Input: part model. Units: mm. Frame: model coordinates. Face numbers are marked on the shaded views. A direction names the side the tool comes from. Give positions to 0.01 mm unless a question says otherwise; leave off trailing zeros. Order: outer loops, then holes, each group sorted by start corner. A loop starts at its lowest first (then second) coordinate and runs counter-clockwise, first axis right, second up.
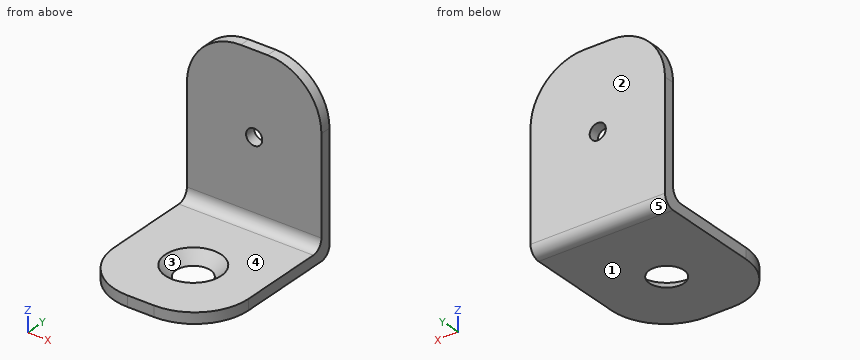
```python
from build123d import *

# Parameters (mm, degrees)
EXTRUDE_1_DEPTH     = 2
EXTRUDE_2_DEPTH     = 2
FILLET_1_R          = 2
FILLET_2_R          = 2
SKETCH_8_R          = 1.5
CUT_EXTRUDE_1_DEPTH = 10


with BuildPart() as part:
    # Эскиз1 → Бобышка-Вытянуть1 (new body)
    with BuildSketch(Plane(origin=(0, 0, 0), x_dir=(1, 0, 0), z_dir=(0, 1, 0))):
        with BuildLine():
            Line((-2.5, -15), (2.5, -15))
            ThreePointArc((2.5, -15), (9.571067812, -12.071067812), (12.5, -5))
            Line((12.5, -5), (12.5, 15))
            Line((12.5, 15), (-12.5, 15))
            Line((-12.5, 15), (-12.5, -5))
            ThreePointArc((-12.5, -5), (-9.571067812, -12.071067812), (-2.5, -15))
        make_face()
    extrude(amount=EXTRUDE_1_DEPTH)

    # Эскиз3 → Бобышка-Вытянуть2 (add)
    with BuildSketch(Plane(origin=(0, 0, -15), x_dir=(-1, 0, 0), z_dir=(0, 0, -1))):
        with BuildLine():
            Line((-2.5, -28), (2.5, -28))
            ThreePointArc((2.5, -28), (9.571067812, -25.071067812), (12.5, -18))
            Line((12.5, -18), (12.5, 2))
            Line((12.5, 2), (-12.5, 2))
            Line((-12.5, 2), (-12.5, -18))
            ThreePointArc((-12.5, -18), (-9.571067812, -25.071067812), (-2.5, -28))
        make_face()
    extrude(amount=EXTRUDE_2_DEPTH)

    # Скругление1
    fillet_1_edges = [part.edges().sort_by_distance(p)[0] for p in [
        (0, 0, -15),
    ]]
    fillet(fillet_1_edges, radius=FILLET_1_R)

    # Скругление2
    fillet_2_edges = [part.edges().sort_by_distance(p)[0] for p in [
        (0, 2, -17),
    ]]
    fillet(fillet_2_edges, radius=FILLET_2_R)

    # Эскиз7 → Зенковка для винта с полупотайной головкой M52 (revolve, cut)
    with BuildSketch(Plane(origin=(0, -15.034247801, -15), x_dir=(0, -1, 0), z_dir=(1, 0, 0))):
        Polygon((0, 0), (0, 2), (2.75, 2), (2.75, 2.45), (5.2, 0), align=None)
    revolve(axis=Axis((0, -15.034247801, -8.65), (0, 0, -1)), mode=Mode.SUBTRACT)

    # Эскиз8 → Вырез-Вытянуть1 (cut)
    with BuildSketch(Plane.XZ):
        Circle(SKETCH_8_R)
    extrude(amount=-CUT_EXTRUDE_1_DEPTH, mode=Mode.SUBTRACT)


solid = part.part
```
1) Reachability of the marked faces 4 and 5 from +Z, -Z, +X, -X, +Y, -Y: full face, straight path, thin tool, end or side. Return the list, or none.
2) Cut plane B-B (x = 8.5). Return the cut outline in (y, z), then the cut area to 3 significant figures.
3) Cut plane A-A (z = 0). Return the cut outline in (x, y).
4) Line query: probe 1 along Y at (x, z) = (6.75, 12); probe 2 along Z at (x, y) = (8, -13); probe 3 along Z at (x, y) = (0, 1.2). Output: solid intervals per line, ascending.
5) Cut plane D-D (x = -6). Return the cut outline in (y, z), then the cut area to 3 significant figures.
6) Cut plane C-C (z = -7.5). Return the cut outline in (x, y), then the cut area to 3 significant figures.
7) First-contact query: P1, Ø10, axis at x = 4.5, z = -7, coming from the -Y side; P2, Ø1.8, axis at x = 0, z = 0, coming from the -Y side; P3, Ø12.5, axis at x = 2, y = -18, coming from the +Z side. Flat tips, straight axial feed; report the tip coordinate or a pass-through.
8) Pull-direction query (Y, two-part tool) for the marked faces 1, 2 and 3; classes: pulls with the +Y half, pulls with the -Y half, needs draft (parallel to the pull), parting line crosses it, or undercut.
Geometry says:
1. face 4: +Z, +X, -X, -Y
1. face 5: -Z, +X, -X, +Y
2. outline: (-26, -17) - (0, -17) arc R2 ccw to (2, -15) - (2, 13) - (0, 13) - (0, -13) arc R2 cw to (-2, -15) - (-26, -15) - close
2. area: 112 mm2
3. outline: (-12.5, 0) - (-1.5, 0) - (-1.5, 2) - (-12.5, 2) - close; (1.5, 0) - (12.5, 0) - (12.5, 2) - (1.5, 2) - close
4. probe 1: y = 0 to 2
4. probe 2: z = -17 to -15
4. probe 3: z = -16.6 to -1.5, 1.5 to 15
5. outline: (-27.37, -17) - (0, -17) arc R2 ccw to (2, -15) - (2, 14.37) - (0, 14.37) - (0, -13) arc R2 cw to (-2, -15) - (-27.37, -15) - close
5. area: 117 mm2
6. outline: (-12.5, 0) - (12.5, 0) - (12.5, 2) - (-12.5, 2) - close
6. area: 50.0 mm2
7. P1: stops at y = 0
7. P2: passes through
7. P3: stops at z = -15
8. face 1: needs draft
8. face 2: pulls with the +Y half
8. face 3: undercut
